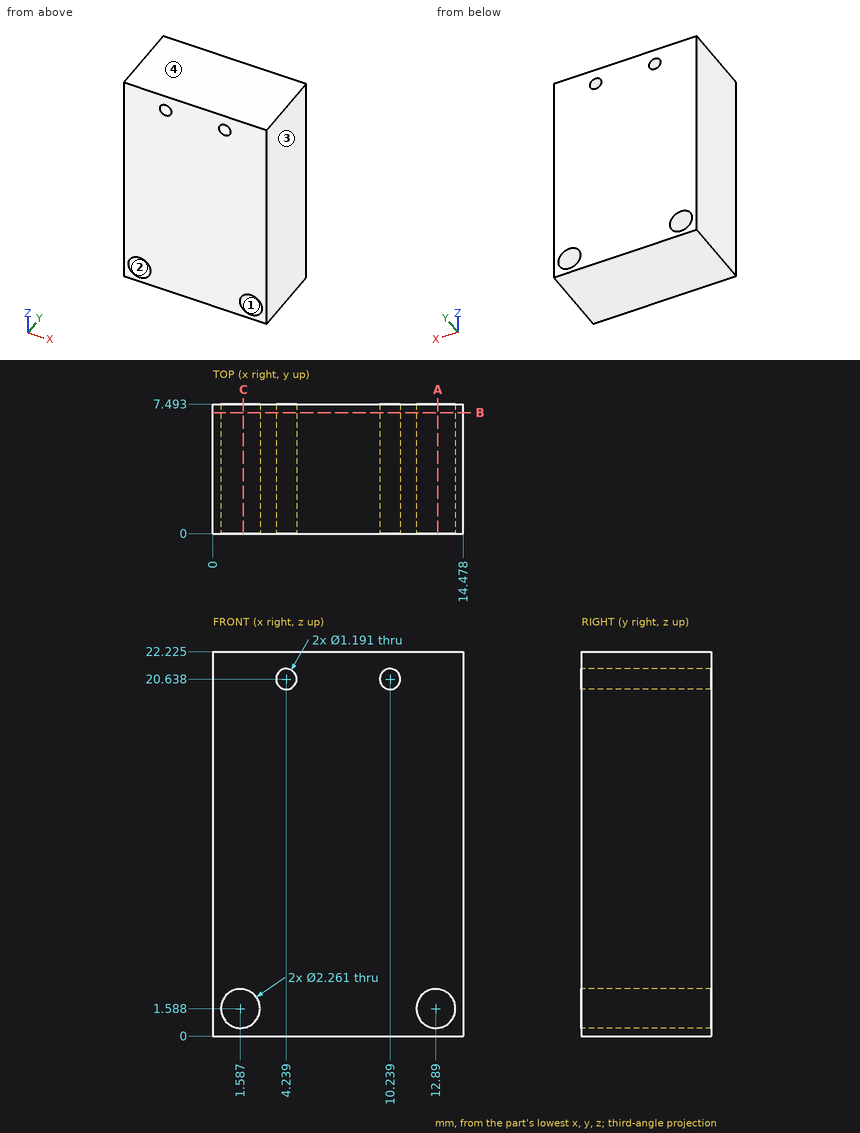
Design review of the part shown in the three views and the two pictorial views. Dimensions are in mm from the part's minimum x, y and z. Round coordinates to 2 decimals unless told otherwise and drop trailing zeros. Write each loop counter-clockwise with the first axis right and the second up, starting at its lowest first coordinate (ties: lowest second). Pieces come first, ordered by that corner, then holes.
1) Take a section at A-A on x = 13. Give the boundary of the cut face in (y, z) (1 decimal), then the cut area to 3 significant figures.
Answer below:
outline: (0, 0) - (7.5, 0) - (7.5, 0.5) - (0, 0.5) - close; (0, 2.7) - (7.5, 2.7) - (7.5, 22.2) - (0, 22.2) - close
area: 150 mm2
2) For line 1 along Z through (x, y) = (13, 5.75) (1 decimal); line 2 along X through (y, z) = (0.5, 1.75) (1 decimal); line 3 along X through (y, z) = (1.5, 2.5) (1 decimal), list the stretches that pass through material, from the lowest coordinate up.
Answer below:
line 1: z = 0 to 0.5, 2.7 to 22.2
line 2: x = 0 to 0.5, 2.7 to 11.8, 14 to 14.5
line 3: x = 0 to 0.9, 2.3 to 12.2, 13.6 to 14.5
3) Insertion check: pin 1 Ø1.1 at (x, z) = (4.24, 20.64) entering from -Y. The pin has a flat end and moves straight along its axis. Give the tip position at first contact, or say it passes through.
Answer below:
pin 1: passes through
4) Take a section at B-B on y = 7. Give the boundary of the cut face in (x, z) (1 decimal).
Answer below:
outline: (0, 0) - (14.5, 0) - (14.5, 22.2) - (0, 22.2) - close; hole circle Ø2.3 at (1.6, 1.6); hole circle Ø1.2 at (4.2, 20.6); hole circle Ø1.2 at (10.2, 20.6); hole circle Ø2.3 at (12.9, 1.6)
5) Mouldability with a two-part tool opening along Z and no side actions: class the marked faces 1, 2, 3 and 4 as +Z half, -Z half, draft (parallel to the pull), parting line (faces both ways), or undercut.
Answer below:
face 1: undercut
face 2: undercut
face 3: draft
face 4: +Z half
